Design review of the part built by this model. Coordinates are the model's own, in mm. A direction names the side the tool comes from. Round coordinates to 2 decimals unless told otherwise and drop trailing zeros. Order: outer loops, then holes, each group sorted by start corner. A loop starts at its lowest first (then second) coordinate and runs counter-clockwise, first axis right, second up.
from build123d import *

# Parameters (mm, degrees)
SKETCH_1_R                   = 20
EXTRUDE_1_DEPTH              = 7
SKETCH_2_R                   = 20.3
EXTRUDE_2_DEPTH              = 1
SKETCH_3_R                   = 6.5
CUT_EXTRUDE_1_DEPTH          = 5
SKETCH_4_R                   = 5.5
CUT_EXTRUDE_2_DEPTH          = 4
CUT_EXTRUDE_START            = -9
SKETCH_5_R                   = 1.5
CUT_EXTRUDE_3_DEPTH          = 10
PATTERN_CIRCULAR_1_COUNT     = 3
HOLE_WIZARD_M3_1_D           = 3.6
HOLE_WIZARD_M3_1_CSINK_D     = 6.3
HOLE_WIZARD_M3_1_CSINK_ANGLE = 90
PATTERN_CIRCULAR_2_COUNT     = 3
M4X0_7_1_D                   = 3.3
M3X0_5_1_D                   = 2.5
PATTERN_CIRCULAR_3_COUNT     = 6


with BuildPart() as part:
    # ｽｹｯﾁ1 → ﾎﾞｽ - 押し出し1 (new body)
    with BuildSketch(Plane.XY):
        Circle(SKETCH_1_R)
    extrude(amount=EXTRUDE_1_DEPTH)

    # ｽｹｯﾁ2 → ﾎﾞｽ - 押し出し2 (add)
    with BuildSketch(Plane.XY.offset(7)):
        Circle(SKETCH_2_R)
    extrude(amount=EXTRUDE_2_DEPTH)

    # ｽｹｯﾁ3 → ｶｯﾄ - 押し出し1 (cut)
    with BuildSketch(Plane.XY.offset(8)):
        Circle(SKETCH_3_R)
    extrude(amount=-CUT_EXTRUDE_1_DEPTH, mode=Mode.SUBTRACT)

    # ｽｹｯﾁ4 → ｶｯﾄ - 押し出し2 (cut, through all)
    with BuildSketch(Plane.XY.offset(3)):
        Circle(SKETCH_4_R)
    extrude(amount=-CUT_EXTRUDE_2_DEPTH, mode=Mode.SUBTRACT)

    # ｽｹｯﾁ5 → ｶｯﾄ - 押し出し3 (cut)
    with BuildSketch(Plane.XY.offset(8).offset(CUT_EXTRUDE_START)):
        with Locations((0, 12)):
            Circle(SKETCH_5_R)
    cut_extrude_3 = extrude(amount=CUT_EXTRUDE_3_DEPTH, mode=Mode.SUBTRACT)

    # 円形ﾊﾟﾀｰﾝ1: ｶｯﾄ - 押し出し3 ×3 about axis
    pattern_circular_1_axis = Axis((0, 0, 0), (0, 0, 1))
    for i in range(1, PATTERN_CIRCULAR_1_COUNT):
        add(cut_extrude_3.rotate(pattern_circular_1_axis, i * 360 / PATTERN_CIRCULAR_1_COUNT), mode=Mode.SUBTRACT)

    # M3 平皿頭ねじ用皿穴1 (through all)
    with Locations(Plane(origin=(0, 0, 0), x_dir=(-1, 0, 0), z_dir=(0, 0, -1))):
        with Locations((0, -14)):
            hole_wizard_m3_1 = CounterSinkHole(HOLE_WIZARD_M3_1_D / 2, HOLE_WIZARD_M3_1_CSINK_D / 2, counter_sink_angle=HOLE_WIZARD_M3_1_CSINK_ANGLE)

    # 円形ﾊﾟﾀｰﾝ2: M3 平皿頭ねじ用皿穴1 ×3 about axis
    pattern_circular_2_axis = Axis((0, 0, 0), (0, 0, 1))
    for i in range(1, PATTERN_CIRCULAR_2_COUNT):
        add(hole_wizard_m3_1.rotate(pattern_circular_2_axis, i * 360 / PATTERN_CIRCULAR_2_COUNT), mode=Mode.SUBTRACT)

    # M4x0.7 ねじ穴1 (through all)
    with Locations(Plane(origin=(0, 0, 0), x_dir=(-1, 0, 0), z_dir=(0, 0, -1))):
        with Locations((15, 0)):
            m4x0_7_1 = Hole(M4X0_7_1_D / 2)

    # M3x0.5 ねじ穴1 (through all)
    with Locations(Plane(origin=(0, 0, 0), x_dir=(-1, 0, 0), z_dir=(0, 0, -1))):
        with Locations((8.5, 0)):
            m3x0_5_1 = Hole(M3X0_5_1_D / 2)

    # 円形ﾊﾟﾀｰﾝ3: M4x0.7 ねじ穴1, M3x0.5 ねじ穴1 ×6 about axis
    pattern_circular_3_axis = Axis((0, 0, 0), (0, 0, 1))
    for i in range(1, PATTERN_CIRCULAR_3_COUNT):
        add(m4x0_7_1.rotate(pattern_circular_3_axis, i * 360 / PATTERN_CIRCULAR_3_COUNT), mode=Mode.SUBTRACT)
        add(m3x0_5_1.rotate(pattern_circular_3_axis, i * 360 / PATTERN_CIRCULAR_3_COUNT), mode=Mode.SUBTRACT)


solid = part.part
1) Take a section at A-A on x = -4.25. Give the boundary of the cut face in (y, z).
Results:
outline: (-19.85, 7) - (-19.54, 7) - (-19.54, 0) - (-8.61, 0) - (-8.61, 8) - (-19.85, 8) - close; (-6.11, 0) - (-3.49, 0) - (-3.49, 3) - (-4.92, 3) - (-4.92, 8) - (-6.11, 8) - close; (3.49, 0) - (6.11, 0) - (6.11, 8) - (4.92, 8) - (4.92, 3) - (3.49, 3) - close; (8.61, 0) - (19.54, 0) - (19.54, 7) - (19.85, 7) - (19.85, 8) - (8.61, 8) - close
2) To check wall thickness, follow line 1 along Y through (x, z) = (0, 6.5); line 2 along Y through (x, z) = (-7.5, 3.25); line 3 along X through (y, z) = (12, 4.75). State the ranges of each line that lie inside material, in increasing order.
Results:
line 1: y = -20 to -15.8, -12.2 to -6.5, 6.5 to 10.5, 13.5 to 20
line 2: y = -18.54 to -14.64, -11.34 to -0.75, 0.75 to 11.34, 14.64 to 18.54
line 3: x = -16 to -8.82, -6.18 to -1.5, 1.5 to 6.18, 8.82 to 16
3) Take a section at B-B on y = 0. State how many separate pieces and enclosed holes the cut face has, plus the area to 3 significant figures.
Results:
separate pieces: 6
enclosed holes: 0
area: 130 mm2
4) For faces 3 (the face through (-5, 3, 3)), 4 (the face through (-9.074, -13.486, 4.056)), list the 3-axis set-ups (+Z, -Z, +X, -X, +Y, -Y) from which the entire face can be reached by the end or side of a thin tool; tool diameter is ignored.
Results:
face 3: +Z
face 4: +Z, -Z
5) Clearance check with flat-ended pins moving along their axes: P1, Ø1.5, axis at x = -12, z = 2, coming from the +Y side; P2, Ø2, axis at x = 4.25, y = 7.36, coming from the +Z side; P3, Ø1.5, axis at y = -1, z = 7, coming from the -X side; P4, Ø3, axis at x = -0.5, z = 3, coming from the +Y side. State where each tip first meets the part, or that it passes through.
Results:
P1: stops at y = 16.54
P2: passes through
P3: stops at x = -20.3
P4: stops at y = 20
6) The part is to be moulded in two halves that separate along Y. For faces 1 (the face through (-4.336, -19.524, 3.451)), 2 (the face through (-11.89, -5.93, 3.94)), say which applies: released by +Y, released by -Y, zero draft, split by the parting line, or undercut.
Results:
face 1: split by the parting line
face 2: undercut
7) Take a section at D-D on y = -8. Give the boundary of the cut face in (x, z), plus the area to 3 significant figures.
Results:
outline: (-18.66, 7) - (-18.33, 7) - (-18.33, 0) - (-5.32, 0) - (-5.32, 8) - (-18.66, 8) - close; (-3.18, 0) - (3.18, 0) - (3.18, 8) - (-3.18, 8) - close; (5.32, 0) - (18.33, 0) - (18.33, 7) - (18.66, 7) - (18.66, 8) - (5.32, 8) - close
area: 260 mm2
